from build123d import *


with BuildPart() as part:
    # Sketch2 → Revolve1 (revolve)
    with BuildSketch(Plane(origin=(0, 0, 0), x_dir=(0, 0, -1), z_dir=(1, 0, 0))):
        with BuildLine():
            Line((-1.5875, -2.778125), (-1.5875, 2.778125))
            Line((-1.5875, 2.778125), (-3.175, 2.778125))
            ThreePointArc((-3.175, 2.778125), (-4.26188695, 2.073570621), (-4.062439479, 0.79375))
            Line((-4.062439479, 0.79375), (-3.175, 0.79375))
            Line((-3.175, 0.79375), (-3.175, -0.79375))
            Line((-3.175, -0.79375), (-4.062439479, -0.79375))
            ThreePointArc((-4.062439479, -0.79375), (-4.26188695, -2.073570621), (-3.175, -2.778125))
            Line((-3.175, -2.778125), (-1.5875, -2.778125))
        make_face()
    revolve(axis=Axis((0, -2.778125, 0), (0, 1, 0)))


solid = part.part
For this review, take the finished solid that the model builds, in its own axes (mm). A direction names the side the tool comes from. Give positions to 0.01 mm unless a question says otherwise; leave off trailing zeros. Loops run counter-clockwise (first coordinate to the right, second up) from the corner with the lowest first, then second, coordinate; pieces in that order, holes last.
Item 1: Take a section at A-A, the plane x = 0. State the section outline as (y, z) points (1 decimal), and give its area (3 significant figures).
Item 2: For line 1 along X through (y, z) = (0.05, 0) (1 decimal); line 2 along X through (y, z) = (0.9, 0); line 3 along Y through (x, z) = (0.5, -3.25), list the stretches that pass through material, from the lowest coordinate up.
Item 3: Take a section at D-D, the plane y = -1.15. State the section outline as (x, z) points (1 decimal), and give its area (3 significant figures).
Item 4: Draft analysis for pull direction Z (two halves, no side actions). For faces 3 (the cylindrical face through (-1.55, 0.04, -0.34)), 4 (the cylindrical face through (-3.1, -0.01, -0.69)), 5 (the flat face through (-3, -0.794, -2)), state which applies: +Z half, -Z half, draft (parallel to the pull), parting line (faces both ways), or undercut.
Item 5: Take a section at B-B, the plane z = 0. State the section outline as (x, y) points (1 decimal), and give its area (3 significant figures).
Item 6: Insertion check: pin 1 (3 mm diameter, centred on x = 3, y = -1, fed in from +Z); pin 2 (3 mm diameter, centred on y = 0, z = 1, fed in from -X); pin 3 (1.5 mm diameter, centred on x = -1.5, y = -2, fed in from -Z); pin 4 (3 mm diameter, centred on x = 0, z = 0, fed in from -Y). Each pin has a flat end and moves straight along its axis. Give the tip position at first contact, or say it passes through.
Item 7: Tool access review of faces 1 (the flat face through (-3, 0.794, 2)), 2 (the flat face through (-1.4, 2.778, -1.4)): name each direction out of +Z, -Z, +X, -X, +Y, -Y from which nothing blocks a thin tool from reaching the whole face with its end or side.
Calculated:
1. outline: (-2.8, -3.2) arc R1.2 ccw to (-0.8, -4.1) - (-0.8, -3.2) - (0.8, -3.2) - (0.8, -4.1) arc R1.2 ccw to (2.8, -3.2) - (2.8, -1.6) - (-2.8, -1.6) - close; (-2.8, 1.6) - (2.8, 1.6) - (2.8, 3.2) arc R1.2 ccw to (0.8, 4.1) - (0.8, 3.2) - (-0.8, 3.2) - (-0.8, 4.1) arc R1.2 ccw to (-2.8, 3.2) - close
1. area: 25.6 mm2
2. line 1: x = -3.2 to -1.6, 1.6 to 3.2
2. line 2: x = -4.15 to -1.59, 1.59 to 4.15
2. line 3: y = -2.77 to -0.79, 0.79 to 2.77
3. outline: circle Ø8.6 at (0, 0); hole circle Ø3.2 at (0, 0)
3. area: 49.7 mm2
4. face 3: undercut
4. face 4: parting line
4. face 5: draft
5. outline: (-4.1, -0.8) arc R1.2 ccw to (-3.2, -2.8) - (-1.6, -2.8) - (-1.6, 2.8) - (-3.2, 2.8) arc R1.2 ccw to (-4.1, 0.8) - (-3.2, 0.8) - (-3.2, -0.8) - close; (1.6, -2.8) - (3.2, -2.8) arc R1.2 ccw to (4.1, -0.8) - (3.2, -0.8) - (3.2, 0.8) - (4.1, 0.8) arc R1.2 ccw to (3.2, 2.8) - (1.6, 2.8) - close
5. area: 25.6 mm2
6. pin 1: stops at z = 4.07
6. pin 2: stops at x = -4.33
6. pin 3: stops at z = -4.28
6. pin 4: passes through
7. face 1: none
7. face 2: +Z, -Z, +X, -X, +Y
